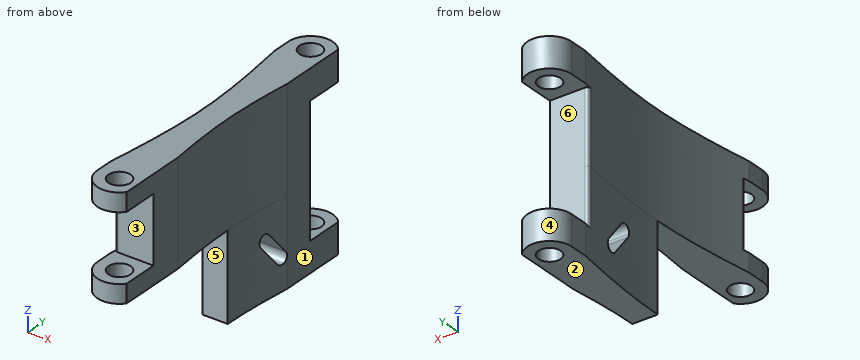
```python
from build123d import *

# Parameters (mm, degrees)
F0_R     = 1.75
F1_DEPTH = 16.3
F2_W     = 0.6277186767
F2_H     = 10.5
F2_W_2   = 2.8722813233
F2_W_3   = 3.5
F3_DEPTH = 25
F4_DEPTH = 13.7
F5_W     = 3.75
F5_H     = 20.5
F6_DEPTH = 25
F7_R     = 0.5
F9_DEPTH = 44


# Not quite as in the source:
# - a feature names something its author has since deleted; it is built from what else it names


with BuildPart() as f1:
    # F0 (on Top) → F1 (new body)
    with BuildSketch(Plane.XY):
        with BuildLine():
            ThreePointArc((-3.5, 0), (0, -3.5), (3.5, 0))
            ThreePointArc((3.5, 0), (0, 3.5), (-3.5, 0))
        make_face()
        Circle(F0_R, mode=Mode.SUBTRACT)
        with BuildLine():
            ThreePointArc((-3.5, 40.5), (0, 37), (3.5, 40.5))
            ThreePointArc((3.5, 40.5), (0, 44), (-3.5, 40.5))
        make_face()
        with Locations((0, 40.5)):
            Circle(F0_R, mode=Mode.SUBTRACT)
        with BuildLine():
            Line((-2, 20.25), (2, 20.25))
            add(Edge.make_bspline(
                [(3.5, 37.6277186767), (2.75, 32.25), (2, 26.25), (2, 20.25)],
                knots=[0, 0, 0, 0, 0.5, 0.5, 0.5, 0.5], degree=3))
            Line((3.5, 37.6277186767), (3.5, 40.5))
            ThreePointArc((3.5, 40.5), (0, 37), (-3.5, 40.5))
            Line((-3.5, 40.5), (-3.5, 37.6277186767))
            add(Edge.make_bspline(
                [(-3.5, 37.6277186767), (-2.75, 32.25), (-2, 26.25), (-2, 20.25)],
                knots=[0, 0, 0, 0, 0.5, 0.5, 0.5, 0.5], degree=3))
        make_face()
        with BuildLine():
            ThreePointArc((-3.5, 0), (0, 3.5), (3.5, 0))
            Line((3.5, 0), (3.5, 2.8722813233))
            add(Edge.make_bspline(
                [(2, 20.25), (2, 14.25), (2.75, 8.25), (3.5, 2.8722813233)],
                knots=[0.5, 0.5, 0.5, 0.5, 1, 1, 1, 1], degree=3))
            Line((2, 20.25), (-2, 20.25))
            add(Edge.make_bspline(
                [(-2, 20.25), (-2, 14.25), (-2.75, 8.25), (-3.5, 2.8722813233)],
                knots=[0.5, 0.5, 0.5, 0.5, 1, 1, 1, 1], degree=3))
            Line((-3.5, 2.8722813233), (-3.5, 0))
        make_face()
    extrude(amount=F1_DEPTH)

    # F2 (on face) → F3 (cut)
    with BuildSketch(Plane(origin=(-3.5, 0, 0), x_dir=(0, -1, 0), z_dir=(-1, 0, 0))):
        with Locations((-3.1861406616, 8.15)):
            Rectangle(F2_W, F2_H)
        with Locations((-1.4361406616, 8.15)):
            Rectangle(F2_W_2, F2_H)
        with Locations((1.75, 8.15)):
            Rectangle(F2_W_3, F2_H)
    extrude(amount=-F3_DEPTH, mode=Mode.SUBTRACT)

    # F0 (on Top) → F4 (join)
    with BuildSketch(Plane.XY):
        with BuildLine():
            ThreePointArc((-3.5, 40.5), (0, 37), (3.5, 40.5))
            ThreePointArc((3.5, 40.5), (0, 44), (-3.5, 40.5))
        make_face()
        with Locations((0, 40.5)):
            Circle(F0_R, mode=Mode.SUBTRACT)
        with BuildLine():
            Line((-2, 20.25), (2, 20.25))
            add(Edge.make_bspline(
                [(3.5, 37.6277186767), (2.75, 32.25), (2, 26.25), (2, 20.25)],
                knots=[0, 0, 0, 0, 0.5, 0.5, 0.5, 0.5], degree=3))
            Line((3.5, 37.6277186767), (3.5, 40.5))
            ThreePointArc((3.5, 40.5), (0, 37), (-3.5, 40.5))
            Line((-3.5, 40.5), (-3.5, 37.6277186767))
            add(Edge.make_bspline(
                [(-3.5, 37.6277186767), (-2.75, 32.25), (-2, 26.25), (-2, 20.25)],
                knots=[0, 0, 0, 0, 0.5, 0.5, 0.5, 0.5], degree=3))
        make_face()
    extrude(amount=-F4_DEPTH)

    # F5 (on face) → F6 (cut)
    with BuildSketch(Plane(origin=(-3.5, 0, 0), x_dir=(0, -1, 0), z_dir=(-1, 0, 0))):
        with Locations((-42.375, 1.3)):
            Rectangle(F5_W, F5_H)
        Polygon((-37.6277186767, 0), (-37.6277186767, 11.55), (-40.5, 11.55), (-40.5, -8.95), (-37.6277186767, -8.95), align=None)
        Polygon((-36.75, -8.95), (-36.75, 11.55), (-37.6277186767, 11.55), (-37.6277186767, 0), (-37.6277186767, -8.95), align=None)
        with BuildLine():
            ThreePointArc((-30.0909245811, -9.4078987175), (-29.9172764034, -9.1071312511), (-29.8569690242, -8.7651111078))
            ThreePointArc((-29.8569690242, -8.7651111078), (-30.5149488809, -7.825418487), (-31.6230134673, -8.1223234981))
            ThreePointArc((-31.6230134673, -8.1223234981), (-31.4997566339, -9.5311555509), (-30.0909245811, -9.4078987175))
        make_face()
        with BuildLine():
            ThreePointArc((-31.6230134673, -8.1223234981), (-30.5149488809, -7.825418487), (-29.8569690242, -8.7651111078))
            ThreePointArc((-29.8569690242, -8.7651111078), (-29.9172764034, -9.1071312511), (-30.0909245811, -9.4078987175))
            Line((-30.0909245811, -9.4078987175), (-26.8769865327, -5.5776765019))
            ThreePointArc((-26.8769865327, -5.5776765019), (-28.2858185855, -5.7009333353), (-28.4090754189, -4.2921012825))
            Line((-28.4090754189, -4.2921012825), (-31.6230134673, -8.1223234981))
        make_face()
        with BuildLine():
            ThreePointArc((-26.6430309758, -4.9348888922), (-27.3010108325, -3.9951962714), (-28.4090754189, -4.2921012825))
            ThreePointArc((-28.4090754189, -4.2921012825), (-28.2858185855, -5.7009333353), (-26.8769865327, -5.5776765019))
            ThreePointArc((-26.8769865327, -5.5776765019), (-26.703338355, -5.2769090355), (-26.6430309758, -4.9348888922))
        make_face()
    extrude(amount=-F6_DEPTH, mode=Mode.SUBTRACT)

    # F7
    f7_edges = [f1.edges().sort_by_distance(p)[0] for p in [
        (-3.412885, 3.5, 8.15),
        (3.412885, 3.5, 8.15),
        (3.378456, 36.75, 5.775),
        (3.378456, 36.75, -4.475),
        (-3.378456, 36.75, 5.775),
        (-3.378456, 36.75, -4.475),
    ]]
    fillet(f7_edges, radius=F7_R)

    # F8 (on face) → F9 (cut)
    with BuildSketch(Plane.XY.offset(16.3)):
        with BuildLine():
            ThreePointArc((3.5, 40.5), (3.3071891388, 41.6456439237), (2.75, 42.6650635095))
            Line((2.75, 42.6650635095), (2.75, 31.8256302364))
            add(Edge.make_bspline(
                [(2.75, 31.8256302364), (2.979055467, 33.8173381724), (3.2395277335, 35.7600565803), (3.5, 37.6277186767)],
                knots=[1.3263518223, 1.3263518223, 1.3263518223, 1.3263518223, 1.5, 1.5, 1.5, 1.5], degree=3))
            Line((3.5, 37.6277186767), (3.5, 40.5))
        make_face()
        with BuildLine():
            add(Edge.make_bspline(
                [(3.5, 2.8722813233), (3.2395277335, 4.7399434197), (2.979055467, 6.6826618276), (2.75, 8.6743697636)],
                knots=[0.5, 0.5, 0.5, 0.5, 0.6736481777, 0.6736481777, 0.6736481777, 0.6736481777], degree=3))
            Line((2.75, 8.6743697636), (2.75, -2.1650635095))
            ThreePointArc((2.75, -2.1650635095), (3.3071891388, -1.1456439237), (3.5, 0))
            Line((3.5, 0), (3.5, 2.8722813233))
        make_face()
    extrude(amount=-F9_DEPTH, mode=Mode.SUBTRACT)


solid = f1.part
```
For this review, take the finished solid that the model builds, in its own axes (mm). Face numbers are marked on the shaded views. A direction names the side the tool comes from. Coordinates: 2 decimals unless noted, no trailing zeros. Order: outer loops, then holes, each group sorted by start corner. A loop starts at its lowest first (then second) coordinate and runs counter-clockwise, first axis right, second up. Notation, with made-up numbers: (80.5, -16) -> (108.5, -16) arc R13 cw to (108.5, 0) -> close; hole circle Ø10 at (6, 28). An arc over 180 degrees is marked (long way). Use CSV: the item, a comma, the result in double quotes. Start each with the question number.
Item 1: We need section A-A, the plane x = 0. Give the number of separate pieces and of enclosed holes in the cut face, then the cut area to 3 significant figures.
Item 2: Draft analysis for pull direction Z (two halves, no side actions). For the marked faces 1, 2 and 3, state which applies: pulls with the +Z half, pulls with the -Z half, needs draft (parallel to the pull), parting line crosses it, or undercut.
Item 3: We need section B-B, the plane y = 40. Give the boundary of the cut face in (x, z).
Item 4: Wall thickness on probe 1 along Y at (x, z) = (0, 14.7); probe 2 along Y at (x, z) = (0, -10.55); probe 3 along X at (y, z) = (0, 1.95): over which ranges is each line inside the solid? List them lowest first.
Item 5: Insertion check: pin 1 (1.9 mm diameter, centred on x = -1, y = 12, fed in from -Z); pin 2 (1 mm diameter, centred on x = -3, z = 6.5, fed in from -Y); pin 3 (4 mm diameter, centred on y = 39, z = 2.5, fed in from +X); pin 4 (1.2 mm diameter, centred on x = 0, z = -5, fed in from -Y). Each pin has a flat end and moves straight along its axis. Give the tip position at first contact, or say it passes through.
Item 6: For the marked faces 4, 5 and 6, list the 3-axis set-ups (+Z, -Z, +X, -X, +Y, -Y) from which the entire face can be reached by the end or side of a thin tool; tool diameter is ignored.
Derived:
1,separate pieces,"5"
1,enclosed holes,"1"
1,area,"811 mm^2"
2,face 1,"needs draft"
2,face 2,"pulls with the -Z half"
2,face 3,"undercut"
3,outline,"(-3.5, -13.7) -> (-1.68, -13.7) -> (-1.68, -8.95) -> (-3.5, -8.95) -> close; (-3.5, 11.55) -> (-1.68, 11.55) -> (-1.68, 16.3) -> (-3.5, 16.3) -> close; (1.68, -13.7) -> (2.75, -13.7) -> (2.75, -8.95) -> (1.68, -8.95) -> close; (1.68, 11.55) -> (2.75, 11.55) -> (2.75, 16.3) -> (1.68, 16.3) -> close"
4,probe 1,"y = -3.5 to -1.75, 1.75 to 38.75, 42.25 to 44"
4,probe 2,"y = 20.25 to 38.75, 42.25 to 44"
4,probe 3,"x = -3.5 to -1.75, 1.75 to 2.75"
5,pin 1,"stops at z = 0"
5,pin 2,"stops at y = 3.5"
5,pin 3,"passes through"
5,pin 4,"stops at y = 20.25"
6,face 4,"+Z, -Z, +Y"
6,face 5,"-Z, +X, -X, -Y"
6,face 6,"+X, -X, +Y"
